from build123d import *

# Parameters (mm, degrees)
IZIM1_R                      = 19.054564863
Y_KSEKLIK_EKSTR_ZYON1_DEPTH  = 3
IZIM1_3_R                    = 8.05
IZIM1_3_R_2                  = 6.05
Y_KSEKLIK_EKSTR_ZYON2_DEPTH  = 18
Y_KSEKLIK_EKSTR_ZYON10_DEPTH = 18
KES_EKSTR_ZYON1_DEPTH        = 20.054564863
KES_EKSTR_ZYON1_DEPTH_BACK   = 20.054564863
IZIM6_R                      = 1
KES_EKSTR_ZYON2_DEPTH        = 20.054564863
KES_EKSTR_ZYON2_DEPTH_BACK   = 20.054564863


with BuildPart() as part:
    # Çizim1 → Yükseklik-Ekstrüzyon1 (new body)
    with BuildSketch(Plane(origin=(0, 0, 0), x_dir=(1, 0, 0), z_dir=(0, 1, 0))):
        Circle(IZIM1_R)
    extrude(amount=Y_KSEKLIK_EKSTR_ZYON1_DEPTH)

    # Çizim1<3> → Yükseklik-Ekstrüzyon2 (add)
    with BuildSketch(Plane(origin=(0, 0, 0), x_dir=(1, 0, 0), z_dir=(0, 1, 0))):
        Circle(IZIM1_3_R)
        Circle(IZIM1_3_R_2, mode=Mode.SUBTRACT)
    extrude(amount=Y_KSEKLIK_EKSTR_ZYON2_DEPTH)

    # Çizim1<11> → Yükseklik-Ekstrüzyon10 (add)
    with BuildSketch(Plane(origin=(0, 0, 0), x_dir=(1, 0, 0), z_dir=(0, 1, 0))):
        with BuildLine():
            ThreePointArc((-7.952358141, -1.25), (-8.05, 0), (-7.952358141, 1.25))
            Line((-7.952358141, 1.25), (-13.952358141, 1.25))
            Line((-13.952358141, 1.25), (-13.952358141, -1.25))
            Line((-13.952358141, -1.25), (-7.952358141, -1.25))
        make_face()
        with BuildLine():
            Line((13.952358141, 1.25), (7.952358141, 1.25))
            ThreePointArc((7.952358141, 1.25), (8.025552412, 0.626903887), (8.05, 0))
            ThreePointArc((8.05, 0), (8.025552412, -0.626903887), (7.952358141, -1.25))
            Line((7.952358141, -1.25), (13.952358141, -1.25))
            Line((13.952358141, -1.25), (13.952358141, 1.25))
        make_face()
    extrude(amount=Y_KSEKLIK_EKSTR_ZYON10_DEPTH)

    # Çizim5 → Kes-Ekstrüzyon1 (cut, two sides)
    with BuildSketch(Plane.XY) as kes_ekstr_zyon1_sk:
        Polygon((-13.952358141, 3), (-7.952358141, 18), (-13.952358141, 18), align=None)
        Polygon((7.952358141, 18), (13.952358141, 18), (13.952358141, 3), align=None)
    extrude(amount=KES_EKSTR_ZYON1_DEPTH, mode=Mode.SUBTRACT)
    extrude(kes_ekstr_zyon1_sk.sketch, amount=-KES_EKSTR_ZYON1_DEPTH_BACK, mode=Mode.SUBTRACT)

    # Çizim6 → Kes-Ekstrüzyon2 (cut, two sides)
    with BuildSketch(Plane.XY) as kes_ekstr_zyon2_sk:
        with Locations((0, 11)):
            Circle(IZIM6_R)
    extrude(amount=KES_EKSTR_ZYON2_DEPTH, mode=Mode.SUBTRACT)
    extrude(kes_ekstr_zyon2_sk.sketch, amount=-KES_EKSTR_ZYON2_DEPTH_BACK, mode=Mode.SUBTRACT)


solid = part.part
Geometry check sheet. Reference: the model listing, model coordinates, mm. A direction names the side the tool comes from. Give positions to 0.01 mm unless a question says otherwise; leave off trailing zeros. Order: outer loops, then holes, each group sorted by start corner. A loop starts at its lowest first (then second) coordinate and runs counter-clockwise, first axis right, second up. Notation, with made-up numbers: (-31.75, 23.5) - (26.25, 23.5) arc R14 ccw to (26.25, 28.5) - close; hole circle Ø1 at (-34.75, 57.5). An arc over 180 degrees is marked (long way). Answer as a JSON object with one key per item and string values.
(1) Cross-section at A-A (x = 0). Record the cut outline in (y, z).
Report:
{"outline": "(0, -19.05) - (3, -19.05) - (3, -8.05) - (10, -8.05) - (10, -6.05) - (3, -6.05) - (3, 6.05) - (10, 6.05) - (10, 8.05) - (3, 8.05) - (3, 19.05) - (0, 19.05) - close; (12, -8.05) - (18, -8.05) - (18, -6.05) - (12, -6.05) - close; (12, 6.05) - (18, 6.05) - (18, 8.05) - (12, 8.05) - close"}
(2) Draft check along Z on faces 4 (the flat face through (-10, 7, 1.25)), 5 (the cylindrical face through (2.79, 10.4, 5.37)), 6 (the flat face through (-10, 9, -1.25)), 7 (the cylindrical face through (0, 10, 7)). Enter one of: released by +Z, released by -Z, zero draft, split by the parting line, or undercut.
Report:
{"face 4": "released by +Z", "face 5": "undercut", "face 6": "released by -Z", "face 7": "zero draft"}
(3) Cross-section at B-B (y = 11). Record the cut outline in (x, z).
Report:
{"outline": "(-10.75, -1.25) - (-7.95, -1.25) arc R8.05 ccw to (-1, -7.99) - (-1, -5.97) arc R6.05 cw to (-1, 5.97) - (-1, 7.99) arc R8.05 ccw to (-7.95, 1.25) - (-10.75, 1.25) - close; (1, -7.99) arc R8.05 ccw to (7.95, -1.25) - (10.75, -1.25) - (10.75, 1.25) - (7.95, 1.25) arc R8.05 ccw to (1, 7.99) - (1, 5.97) arc R6.05 cw to (1, -5.97) - close"}
(4) Cross-section at C-C (y = 7). Record the cut outline in (x, z).
Report:
{"outline": "(-12.35, -1.25) - (-7.95, -1.25) arc R8.05 ccw to (7.95, -1.25) - (12.35, -1.25) - (12.35, 1.25) - (7.95, 1.25) arc R8.05 ccw to (-7.95, 1.25) - (-12.35, 1.25) - close; hole circle Ø12.1 at (0, 0)"}
(5) Cross-section at D-D (z = 0). Record the cut outline in (x, y), then the cut area to 3 significant figures.
Report:
{"outline": "(-19.05, 0) - (19.05, 0) - (19.05, 3) - (13.95, 3) - (7.95, 18) - (6.05, 18) - (6.05, 3) - (-6.05, 3) - (-6.05, 18) - (-7.95, 18) - (-13.95, 3) - (-19.05, 3) - close", "area": "261 mm^2"}
(6) Material ranges on line 1 (Z direction, x = 0, y = 8.5); line 2 (Y direction, x = 0, z = 6.75); line 3 (Z direction, x = -8, y = 16.25), recorded low to high.
Report:
{"line 1": "-8.05 to -6.05, 6.05 to 8.05", "line 2": "0 to 10, 12 to 18", "line 3": "-1.25 to 1.25"}
(7) Depth check by flat-ended pin: pin 1 Ø5 at (x, y) = (-10.5, 9.5) entering from -Z; pin 2 Ø6 at (x, z) = (2.5, 1.5) entering from +Y; pin 3 Ø5 at (x, y) = (-12, 8) entering from +Z. Enter the tip coordinate at first touch or a pass-through.
Report:
{"pin 1": "z = -1.25", "pin 2": "y = 3", "pin 3": "z = 1.25"}
(8) Tool access check on faces 1 (the cylindrical face through (0.16, 8.73, -8.05)), 2 (the flat face through (-0.3, 3, 8.2)), 3 (the cylindrical face through (-0.16, 8.73, 8.05)). Record the directions out of +Z, -Z, +X, -X, +Y, -Y that give a thin tool (end or side, any length) a straight path to the whole face; none if there is none.
Report:
{"face 1": "-Z, +Y", "face 2": "+Y", "face 3": "+Z, +Y"}
